Model file for the job. Use its own axes, mm. A direction names the side the tool comes from. Coordinates: 2 decimals unless noted, no trailing zeros. Order: outer loops, then holes, each group sorted by start corner. A loop starts at its lowest first (then second) coordinate and runs counter-clockwise, first axis right, second up. Notation, with made-up numbers: (9.25, 53) -> (22.25, 53) arc R22 ccw to (22.25, 85) -> close; hole circle Ø9 at (16.25, 66). An arc over 180 degrees is marked (long way). Use CSV: the item, a comma, the result in double quotes. Start each with the question number.
(1) Tool access for faces 1 (the cylindrical face through (-10.54, -12.44, 12.46)), 2 (the flat face through (-10, -10, 15)): list every direction of +Z, -Z, +X, -X, +Y, -Y with a clear straight run to the whole face (end or side of a thin tool).
(2) Cut at C-C on z = 12.5. Write the cut outline in (x, y).
(3) Cut at B-B on x = -10. Write the cut outline in (y, z).
(4) Pin check, flat tips, straight feed: pin 1 Ø6 at (y, z) = (-11.5, 5.5) entering from +X; pin 2 Ø2 at (x, y) = (-17, -12.5) entering from +Z. Stop position of each tip, or through.
(5) Cut at A-A on y = -10. Write the cut outline in (x, z).
(6) Probe L1, parallel to Z at x = -4, y = -14.25; L2, parallel to X at y = -2.5, z = 4.25; L3, parallel to X at y = -1, z = 3.5. List the from-to ranges inside material, lowest first.
(7) Cut at D-D on y = -6.5. Write the cut outline in (x, z), plus the area to 3 significant figures.
```python
from build123d import *

# Parameters (mm, degrees)
F1_DEPTH = 20
F2_R     = 2.5
F3_DEPTH = 15


with BuildPart() as f1:
    # F0 (on Front) → F1 (new body)
    with BuildSketch(Plane.XZ):
        Polygon((-20, 0), (0, 0), (-3.64, 10), (-16.36, 10), align=None)
    extrude(amount=F1_DEPTH)

    # F2 (on Top) → F3 (join)
    with BuildSketch(Plane.XY):
        with Locations((-10, -10)):
            Circle(F2_R)
    extrude(amount=F3_DEPTH)


solid = f1.part
```
Outcome:
1,face 1,"+Z"
1,face 2,"+Z, +X, -X, +Y, -Y"
2,outline,"circle Ø5 at (-10, -10)"
3,outline,"(-20, 0) -> (0, 0) -> (0, 10) -> (-7.5, 10) -> (-7.5, 15) -> (-12.5, 15) -> (-12.5, 10) -> (-20, 10) -> close"
4,pin 1,"x = -0.91"
4,pin 2,"z = 10"
5,outline,"(-20, 0) -> (0, 0) -> (-3.64, 10) -> (-7.5, 10) -> (-7.5, 15) -> (-12.5, 15) -> (-12.5, 10) -> (-16.36, 10) -> close"
6,L1,"0 to 10"
6,L2,"-18.45 to -1.55"
6,L3,"-18.73 to -1.27"
7,outline,"(-20, 0) -> (0, 0) -> (-3.64, 10) -> (-16.36, 10) -> close"
7,area,"164 mm2"
